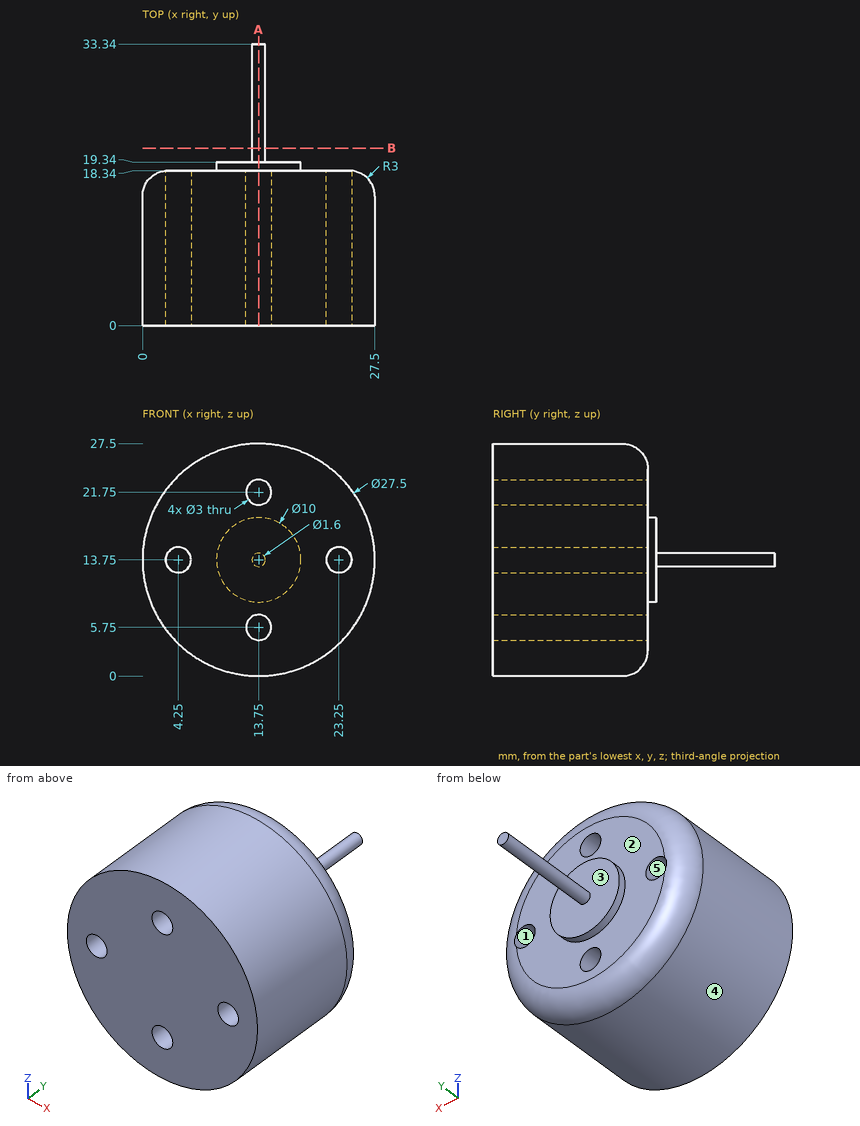
Verification items for this drawing (mm, ordinates from the low corner). A direction names the side the tool comes from. Give positions to 0.01 mm unless a question says otherwise; leave off trailing zeros. Write each loop counter-clockwise with the first axis right and the second up, starting at its lowest first coordinate (ties: lowest second). Pieces come first, ordered by that corner, then holes.
1) Release check for a two-part mould opening along X. For the marked faces 3, 4 and 5 record: released by +X, released by -X, zero draft, split by the parting line, or undercut.
Values follow:
face 3: zero draft
face 4: split by the parting line
face 5: undercut
2) Go/stop test with flat-tipped pins: pin 1 Ø6 at (x, y) = (22, 6.5) entering from +Z; pin 2 Ø5 at (x, z) = (22, 15.5) entering from +Y; pin 3 Ø5 at (y, z) = (17, 3.5) entering from -X; pin 4 Ø11 at (x, z) = (12.5, 12) entering from +Y. Record where each tip stops, or that it passes through.
Values follow:
pin 1: stops at z = 26.46
pin 2: stops at y = 18.34
pin 3: stops at x = 2.63
pin 4: stops at y = 33.34
3) Set-up check for the marked faces 1 and 2: record each of +Z, -Z, +X, -X, +Y, -Y from which the full face is reachable in a straight line by a thin tool's end or side.
Values follow:
face 1: +Y, -Y
face 2: +Y
4) Cross-section at B-B (y = 21). Record the boundary of the cut face in (x, z), plus the area to 3 significant figures.
Values follow:
outline: circle Ø1.6 at (13.75, 13.75)
area: 2.01 mm2
5) Cross-section at A-A (x = 13.75). Count the separate pieces of the cut face and the enclosed holes in it, plus the area to 3 significant figures.
Values follow:
separate pieces: 3
enclosed holes: 0
area: 423 mm2
6) Thickness scan on line 1 (Z direction, x = 13.75, y = 7.25); line 2 (Y direction, x = 15.5, z = 17.5); line 3 (Y direction, x = 16.5, z = 23.75). Record the ranges inside material, lowest first.
Values follow:
line 1: z = 0 to 4.25, 7.25 to 20.25, 23.25 to 27.5
line 2: y = 0 to 19.34
line 3: y = 0 to 18.34
